Input: part model. Units: mm. Frame: model coordinates. Face numbers are marked on the shaded views. A direction names the side the tool comes from. Coordinates: 2 decimals unless noted, no trailing zeros. Use a Markdown table: item, result. Add a question column.
Q1. Set-up query: the marked faces 1 and 2. Return all of +Z, -Z, +X, -X, +Y, -Y with unobstructed straight access to the full face (end or side cutting, diameter ignored); none if empty.
Q2. Pin query (flat end, axial travel): P1, Ø0.7, axis at y = 6.5, z = -4.5, coming from the -X side; P2, Ø1.5, axis at x = 1.5, y = 2.5, coming from the +Z side; P3, Ø0.7, axis at y = 5, z = 1.5, coming from the +X side. Return the tip coordinate at first contact, or that it passes through.
Q3. Mould query, pull axis X, two halves, no side actions, for the marked faces 3 and 4. Classes: released by +X, released by -X, zero draft, split by the parting line, or undercut.
Q4. Material intervals for probe 1 along X at (y, z) = (6, 1); probe 2 along Z at (x, y) = (-0.75, 1); probe 3 along X at (y, z) = (5, -0.75), sorted ascending. Write a range as from..to.
Q5. Section query A-A (y = 1.75). Give the number of separate pieces and of enclosed holes in the cut face, then the cut area to 3 significant figures.
from build123d import *

# Parameters (mm, degrees)
OTHER_START         = 7.189240539
OTHER_2_OUTLINE_W   = 16
OTHER_2_OUTLINE_H   = 16
OTHER_2_DEPTH       = 1.9877561
SKETCH_20_R         = 2.75
EXTRUDE_2_DEPTH     = 6.5
CUT_EXTRUDE_1_DEPTH = 0.5
SKETCH_22_R         = 4
CUT_EXTRUDE_2_DEPTH = 7.5


# Read off the part's stored shape, not the designer's step: 相交2
with BuildPart() as part:
    # 草图4 → Loft 1 section 0
    with BuildSketch(Plane(origin=(0, 8.2, 0), x_dir=(1, 0, 0), z_dir=(0, 1, 0))):
        with BuildLine():
            Line((-5.6, 6.8), (5.6, 6.8))
            Line((5.6, 6.8), (5.6, -5.7))
            Line((5.6, -5.7), (-5.6, -5.7))
            Line((-5.6, -5.7), (-5.6, 6.8))
        make_face()
    # 草图1 → Loft 1 section 1
    with BuildSketch(Plane(origin=(0, 0, 0), x_dir=(1, 0, 0), z_dir=(0, 1, 0))):
        with BuildLine():
            Line((-8.95, -8.9), (8.95, -8.9))
            Line((8.95, -8.9), (8.95, 8.9))
            Line((8.95, 8.9), (-8.95, 8.9))
            Line((-8.95, 8.9), (-8.95, -8.9))
        make_face()
    loft()

    # 相交2 outline → 相交2 (cut)
    with BuildSketch(Plane(origin=(0, 0, 0), x_dir=(1, 0, 0), z_dir=(0, 0.9872752829851917, -0.15902048800865198)).offset(OTHER_START)):
        Rectangle(OTHER_2_OUTLINE_W, OTHER_2_OUTLINE_H)
    extrude(amount=OTHER_2_DEPTH, mode=Mode.SUBTRACT)

    # 草图19 → Loft 1 2 section 0
    with BuildSketch(Plane(origin=(0, 6.132664073, -0.987788564), x_dir=(1, 0, 0), z_dir=(0, 0.9872752829851916, -0.15902048800865207))):
        with BuildLine():
            Line((-4.985089723, 5.299749211), (4.985089723, 5.299749211))
            Line((4.985089723, 5.299749211), (4.287230721, -5.442213697))
            Line((4.287230721, -5.442213697), (-4.287230721, -5.442213697))
            Line((-4.287230721, -5.442213697), (-4.985089723, 5.299749211))
        make_face()
    # 草图8 → Loft 1 2 section 1
    with BuildSketch(Plane.XZ):
        with BuildLine():
            Line((-7.15, 7.2), (7.15, 7.2))
            Line((7.15, 7.2), (7.15, -7.5))
            Line((7.15, -7.5), (-7.15, -7.5))
            Line((-7.15, -7.5), (-7.15, 7.2))
        make_face()
    loft(mode=Mode.SUBTRACT)

    # 草图20 → 凸台-拉伸2 (add)
    with BuildSketch(Plane.XZ):
        with Locations(Location((0, 0, 0), (0, 0, 270))):
            Circle(SKETCH_20_R)
        Polygon((-2.2, 0.8), (-0.8, 0.8), (-0.8, 2.2), (0.8, 2.2), (0.8, 0.8), (2.2, 0.8), (2.2, -0.8), (0.8, -0.8), (0.8, -2.2), (-0.8, -2.2), (-0.8, -0.8), (-2.2, -0.8), align=None, mode=Mode.SUBTRACT)
    extrude(amount=-EXTRUDE_2_DEPTH)

    # 草图21 → 切除-拉伸1 (cut)
    with BuildSketch(Plane(origin=(0, 7.097759487, -1.143236539), x_dir=(1, 0, 0), z_dir=(0, 0.9872752829851916, -0.15902048800865207))):
        with BuildLine():
            Line((-4.075955723, 4.374408411), (-3.05161678, 4.374408411))
            add(Edge.make_bspline(
                [(-3.05161678, 4.374408411), (-3.001598177, 4.37422557), (-2.904339475, 4.373870045), (-2.763152441, 4.368665036), (-2.630787829, 4.361353255), (-2.507581664, 4.350074843), (-2.393003416, 4.336098995), (-2.287386768, 4.319759613), (-2.190702321, 4.299464771), (-2.102553843, 4.275462633), (-2.02069076, 4.248417722), (-1.944052325, 4.218671859), (-1.871820937, 4.185226888), (-1.803585437, 4.149371864), (-1.740597017, 4.107930824), (-1.680956816, 4.065216099), (-1.626276856, 4.018102997), (-1.576276747, 3.968254753), (-1.53138788, 3.915631236), (-1.491980376, 3.861504021), (-1.458087704, 3.806449275), (-1.43097458, 3.749274429), (-1.410270719, 3.690673858), (-1.394505384, 3.630718089), (-1.385098589, 3.56935381), (-1.384133592, 3.527952708), (-1.38364803, 3.50712075)],
                knots=[0, 0, 0, 0, 1.727133696, 3.358326119, 4.878149777, 6.304391432, 7.629726349, 8.863648063, 9.993787461, 11.039234741, 12.016682314, 12.969840003, 13.87620352, 14.764420512, 15.628515143, 16.477592799, 17.296048855, 18.117800747, 18.913499522, 19.681881416, 20.427899323, 21.142662237, 21.862509911, 22.571095379, 23.281012387, 24, 24, 24, 24], degree=3))
            add(Edge.make_bspline(
                [(-1.38364803, 3.50712075), (-1.385412282, 3.468348204), (-1.388910839, 3.391461246), (-1.42095224, 3.279461488), (-1.471320058, 3.173101493), (-1.529107281, 3.090495822), (-1.584691676, 3.028842776), (-1.631123728, 2.983643069), (-1.682562114, 2.940920335), (-1.738589565, 2.900102161), (-1.799873027, 2.862563579), (-1.865299808, 2.826587473), (-1.935344564, 2.793012224), (-1.98417587, 2.77281639), (-2.009048671, 2.762529404)],
                knots=[0, 0, 0, 0, 1.344649222, 2.666474061, 4.014062304, 5.41970358, 6.150026244, 6.896555969, 7.669043806, 8.471425933, 9.302905494, 10.164184025, 11.06490551, 12, 12, 12, 12], degree=3))
            add(Edge.make_bspline(
                [(-2.009048671, 2.762529404), (-1.977920981, 2.754996611), (-1.917306862, 2.740328204), (-1.829559386, 2.715932573), (-1.747632696, 2.689342975), (-1.670272781, 2.664549503), (-1.599588756, 2.635500242), (-1.533515625, 2.608342187), (-1.473506413, 2.578504898), (-1.401750644, 2.538013126), (-1.320454432, 2.484098783), (-1.232731939, 2.412990017), (-1.157794968, 2.334214687), (-1.093935011, 2.249817411), (-1.043468641, 2.160184049), (-1.006060497, 2.066312746), (-0.983696742, 1.968275226), (-0.981102992, 1.901429924), (-0.979801877, 1.867897994)],
                knots=[0, 0, 0, 0, 1.040401352, 2.025945749, 2.957610977, 3.838748948, 4.663524247, 5.439134026, 6.158967321, 6.838896101, 8.114975742, 9.323328772, 10.499359089, 11.638211642, 12.753227844, 13.830378753, 14.911642469, 16, 16, 16, 16], degree=3))
            add(Edge.make_bspline(
                [(-0.979801877, 1.867897994), (-0.981029473, 1.833646659), (-0.983459912, 1.765834667), (-1.006577059, 1.666832464), (-1.041459332, 1.571612689), (-1.09229665, 1.480899499), (-1.157707146, 1.394733239), (-1.235753214, 1.311173804), (-1.329676927, 1.233761622), (-1.435446571, 1.159592435), (-1.553929285, 1.092855208), (-1.682429672, 1.03354565), (-1.821434347, 0.984996199), (-1.969653473, 0.944188002), (-2.12762314, 0.912897118), (-2.295317391, 0.890925288), (-2.472464022, 0.876289135), (-2.593987323, 0.875045113), (-2.656184088, 0.874408411)],
                knots=[0, 0, 0, 0, 0.763794375, 1.512186817, 2.258665885, 3.022620734, 3.824296693, 4.669829699, 5.569978408, 6.537158664, 7.551586153, 8.60252133, 9.69369207, 10.835799672, 12.033384994, 13.286741793, 14.611328995, 16, 16, 16, 16], degree=3))
            Line((-2.656184088, 0.874408411), (-4.075955723, 0.874408411))
            Line((-4.075955723, 0.874408411), (-4.075955723, 4.374408411))
        make_face()
        with BuildLine():
            Line((-3.582365979, 4.015434052), (-3.582365979, 2.89363918))
            Line((-3.582365979, 2.89363918), (-3.274573511, 2.89363918))
            add(Edge.make_bspline(
                [(-3.274573511, 2.89363918), (-3.229234608, 2.894037102), (-3.14182053, 2.894804303), (-3.015329988, 2.897035757), (-2.898263152, 2.903171565), (-2.790415727, 2.909495423), (-2.6919831, 2.919395843), (-2.602964895, 2.931479837), (-2.522737381, 2.944078774), (-2.43017236, 2.965548195), (-2.325916803, 2.996637022), (-2.213810068, 3.045984254), (-2.114923061, 3.104045743), (-2.031417989, 3.172044051), (-1.963132903, 3.246655866), (-1.913980137, 3.327274535), (-1.882872139, 3.412615332), (-1.879120194, 3.471344935), (-1.877237774, 3.500810654)],
                knots=[0, 0, 0, 0, 1.300077838, 2.506569319, 3.626932325, 4.661071425, 5.603901159, 6.462528421, 7.236988455, 7.931124199, 9.1859622, 10.350118682, 11.434989577, 12.463773904, 13.427075439, 14.32002997, 15.157128221, 16, 16, 16, 16], degree=3))
            add(Edge.make_bspline(
                [(-1.877237774, 3.500810654), (-1.878090356, 3.52026362), (-1.879770849, 3.558606611), (-1.891776361, 3.614572779), (-1.912652517, 3.667069895), (-1.94078659, 3.716733169), (-1.977847183, 3.762720595), (-2.023432155, 3.804723671), (-2.076216593, 3.844102145), (-2.137282697, 3.880116871), (-2.20703143, 3.912207698), (-2.286219485, 3.940566317), (-2.375213143, 3.962587503), (-2.473301087, 3.982952277), (-2.581178984, 3.996632495), (-2.698498063, 4.008322574), (-2.825561166, 4.014251811), (-2.913491199, 4.015030452), (-2.959068703, 4.015434052)],
                knots=[0, 0, 0, 0, 0.704770075, 1.389145107, 2.062265897, 2.745067049, 3.450040637, 4.193008615, 4.985718742, 5.832502292, 6.757032351, 7.764250842, 8.87554471, 10.07639704, 11.392709723, 12.81352688, 14.348328909, 16, 16, 16, 16], degree=3))
            Line((-2.959068703, 4.015434052), (-3.582365979, 4.015434052))
        make_face(mode=Mode.SUBTRACT)
        with BuildLine():
            Line((-3.582365979, 2.534664821), (-3.582365979, 1.23338277))
            Line((-3.582365979, 1.23338277), (-2.925414857, 1.23338277))
            add(Edge.make_bspline(
                [(-2.925414857, 1.23338277), (-2.87843879, 1.233762727), (-2.787984434, 1.23449435), (-2.657071337, 1.236961408), (-2.535944574, 1.242321818), (-2.424505301, 1.251162574), (-2.322676057, 1.260268307), (-2.230585111, 1.273130598), (-2.148143507, 1.287369469), (-2.052767711, 1.309568231), (-1.945828922, 1.343476113), (-1.829800232, 1.395799803), (-1.726263469, 1.457063537), (-1.638169932, 1.52937046), (-1.565540416, 1.607250263), (-1.512850304, 1.69077302), (-1.479720256, 1.778095564), (-1.47548575, 1.838182595), (-1.47339162, 1.867897994)],
                knots=[0, 0, 0, 0, 1.29843179, 2.500184008, 3.618878599, 4.648866362, 5.589855277, 6.444005784, 7.218207981, 7.901363496, 9.149526468, 10.311741131, 11.4128985, 12.464137763, 13.451792752, 14.342600541, 15.180350819, 16, 16, 16, 16], degree=3))
            add(Edge.make_bspline(
                [(-1.47339162, 1.867897994), (-1.474057939, 1.886411489), (-1.475384595, 1.923272276), (-1.486301385, 1.977500806), (-1.503895793, 2.030194167), (-1.529359322, 2.080409977), (-1.561622114, 2.129090654), (-1.600943659, 2.175575902), (-1.646816465, 2.221086121), (-1.700338495, 2.263107634), (-1.758970648, 2.304010862), (-1.82377859, 2.341171111), (-1.893956852, 2.374278996), (-1.96876264, 2.405798633), (-2.049273018, 2.432646906), (-2.135127862, 2.4566183), (-2.226255262, 2.476740829), (-2.288984721, 2.487698036), (-2.32104787, 2.493298635)],
                knots=[0, 0, 0, 0, 0.77785496, 1.548726791, 2.316271961, 3.107298279, 3.908573286, 4.766644542, 5.663022547, 6.620650135, 7.623734104, 8.66706768, 9.757067915, 10.884860646, 12.078135655, 13.322666349, 14.631524187, 16, 16, 16, 16], degree=3))
            add(Edge.make_bspline(
                [(-2.32104787, 2.493298635), (-2.346033301, 2.496750191), (-2.400093694, 2.504218241), (-2.488058336, 2.512220196), (-2.588577808, 2.519174973), (-2.701968389, 2.52441673), (-2.827916954, 2.529782033), (-2.96677814, 2.531897127), (-3.1182147, 2.534390125), (-3.223390168, 2.534570849), (-3.27807912, 2.534664821)],
                knots=[0, 0, 0, 0, 0.631419024, 1.366186615, 2.21079442, 3.154006331, 4.208025658, 5.366807578, 6.630797325, 8, 8, 8, 8], degree=3))
            Line((-3.27807912, 2.534664821), (-3.582365979, 2.534664821))
        make_face(mode=Mode.SUBTRACT)
    extrude(amount=-CUT_EXTRUDE_1_DEPTH, mode=Mode.SUBTRACT)

    # 草图22 → 切除-拉伸2 (cut)
    with BuildSketch(Plane.XZ):
        with Locations((0, -9.5)):
            Circle(SKETCH_22_R)
    extrude(amount=-CUT_EXTRUDE_2_DEPTH, mode=Mode.SUBTRACT)


solid = part.part
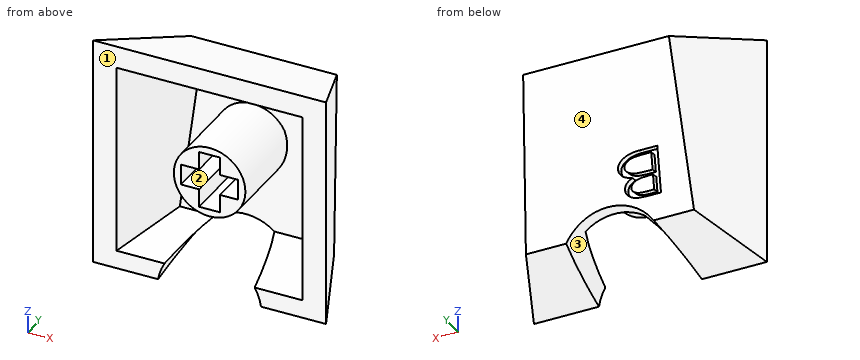
Values follow:
| question | item | result |
|---|---|---|
| 1 | face 1 | +Z, -Z, +X, -X, -Y |
| 1 | face 2 | -Y |
| 2 | P1 | x = -6.44 |
| 2 | P2 | z = 8.22 |
| 2 | P3 | x = 7.05 |
| 3 | face 3 | undercut |
| 3 | face 4 | zero draft |
| 4 | probe 1 | -6.5..-4.7, -2.56..-0.8, 0.8..2.56, 4.7..6.5 |
| 4 | probe 2 | -2.65..-2.2, 2.2..2.65, 6.8..8.51 |
| 4 | probe 3 | -6.91..-5.1, -2.65..-2.2, 2.2..2.65, 5.1..6.91 |
| 5 | separate pieces | 2 |
| 5 | enclosed holes | 1 |
| 5 | area | 102 mm2 |
